Check sheet for the drawn part. Datum: minimum x, y, z corner. Units: mm. A direction names the side the tool comes from. Round coordinates to 2 decimals unless told otherwise and drop trailing zeros. Order: outer loops, then holes, each group sorted by start corner. A loop starts at its lowest first (then second) coordinate and runs counter-clockwise, first axis right, second up. Notation, with made-up numbers: M 13.25,69.25 L 70.25,69.25 A21 cw 70.25,95.25 Z; hole C -39.5,-38.75 d9. An arc over 180 degrees is marked long. Use one line per item in the form item = value. Start each with the question number.
Item 1: Cross-section at D-D on y = 35.5. Enter the section's corners in (x, z), then the cut area to 3 significant figures.
Item 2: Thickness scan on probe 1 along Y at (x, z) = (7, 26.5); probe 2 along Y at (x, z) = (4.25, 21); probe 3 along Z at (x, y) = (1.5, 21) (1 decimal). Record the ranges inside material, lowest first. Write a range as [from, to].
Item 3: Release check for a two-part mould opening along X. For the marked faces 1, 2 and 3 record: +X half, -X half, draft (parallel to the pull), parting line (faces both ways), or undercut.
Item 4: Cross-section at B-B on x = 5.75. Enter the section's corners in (y, z), then the cut area to 3 significant figures.
Item 5: Cross-section at C-C on z = 13.5. Enter the section's corners in (x, y).
Item 6: Cross-section at A-A on y = 20. Enter the section's corners in (x, z), then the cut area to 3 significant figures.
Item 7: Go/stop test with flat-tipped pins: pin 1 Ø1.5 at (x, z) = (5.5, 24.5) entering from -Y; pin 2 Ø3 at (x, z) = (4, 20.5) entering from -Y; pin 3 Ø4 at (x, z) = (7, 22.5) entering from +Y (1 decimal). Record where each tip stops, or that it passes through.
Item 8: Tool access check on the marked faces 4 and 5. Record the directions out of +Z, -Z, +X, -X, +Y, -Y that give a thin tool (end or side, any length) a straight path to the whole face; none if there is none.
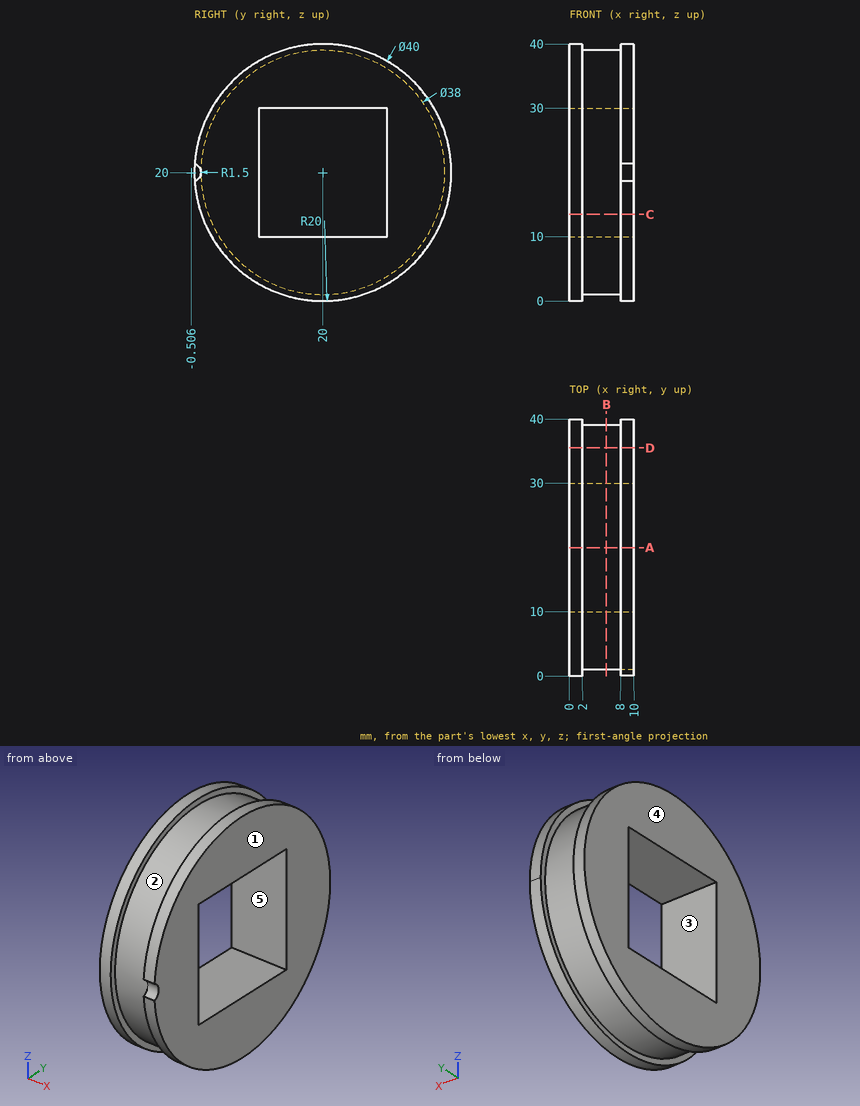
Output values:
q1.outline = M 0,7.36 L 2,7.36 L 2,9.01 L 8,9.01 L 8,7.36 L 10,7.36 L 10,32.64 L 8,32.64 L 8,30.99 L 2,30.99 L 2,32.64 L 0,32.64 Z
q1.area = 233 mm2
q2.probe_1 = [2.15, 10], [30, 37.85]
q2.probe_2 = [1.03, 10], [30, 38.97]
q2.probe_3 = [0, 10], [30, 40]
q3.face_1 = +X half
q3.face_2 = undercut
q3.face_3 = draft
q4.outline = C 20,20 d38; hole M 10,10 L 30,10 L 30,30 L 10,30 Z
q4.area = 734 mm2
q5.outline = M 0,1.09 L 2,1.09 L 2,2.15 L 8,2.15 L 8,1.09 L 10,1.09 L 10,10 L 0,10 Z; M 0,30 L 10,30 L 10,38.91 L 8,38.91 L 8,37.85 L 2,37.85 L 2,38.91 L 0,38.91 Z
q6.outline = M 0,0 L 2,0 L 2,1 L 8,1 L 8,0 L 10,0 L 10,10 L 0,10 Z; M 0,30 L 10,30 L 10,40 L 8,40 L 8,39 L 2,39 L 2,40 L 0,40 Z
q6.area = 188 mm2
q7.pin_1 = 1.37
q7.pin_2 = 1
q7.pin_3 = 40
q8.face_4 = +Z, -Z, -X, +Y, -Y
q8.face_5 = +X, -X
